from build123d import *

# Parameters (mm, degrees)
SKETCH1_W           = 27
SKETCH1_H           = 50
BOSS_EXTRUDE1_DEPTH = 4.5
SKETCH2_W           = 8.18
SKETCH2_H           = 8.18
BOSS_EXTRUDE2_DEPTH = 6.7
SKETCH3_R           = 0.8
CUT_EXTRUDE1_DEPTH  = 6.7


with BuildPart() as part:
    # Sketch1 → Boss-Extrude1 (new body)
    with BuildSketch(Plane.XY):
        Rectangle(SKETCH1_W, SKETCH1_H)
    extrude(amount=BOSS_EXTRUDE1_DEPTH)

    # Sketch2 → Boss-Extrude2 (add)
    with BuildSketch(Plane.XY.offset(4.5)):
        with Locations((0, 18)):
            Rectangle(SKETCH2_W, SKETCH2_H)
    extrude(amount=BOSS_EXTRUDE2_DEPTH)

    # Sketch3 → Cut-Extrude1 (cut)
    with BuildSketch(Plane.XY.offset(4.5)):
        with Locations((10.7092899, 15.271061343)):
            Circle(SKETCH3_R)
        with Locations((10.7092899, 12.271061343)):
            Circle(SKETCH3_R)
        with Locations((10.7092899, 9.271061343)):
            Circle(SKETCH3_R)
        with Locations((10.7092899, 6.271061343)):
            Circle(SKETCH3_R)
        with Locations((10.7092899, 3.271061343)):
            Circle(SKETCH3_R)
        with Locations((10.7092899, 0.271061343)):
            Circle(SKETCH3_R)
        with Locations((10.7092899, -2.728938657)):
            Circle(SKETCH3_R)
        with Locations((10.7092899, -5.728938657)):
            Circle(SKETCH3_R)
        with Locations((10.7092899, -8.728938657)):
            Circle(SKETCH3_R)
        with Locations((10.7092899, -11.728938657)):
            Circle(SKETCH3_R)
    cut_extrude1 = extrude(amount=-CUT_EXTRUDE1_DEPTH, mode=Mode.SUBTRACT)

    # Mirror1: Cut-Extrude1 across plane
    add(cut_extrude1.mirror(Plane(origin=(0, 0, 0), x_dir=(0, 0, 1), z_dir=(1, 0, 0))), mode=Mode.SUBTRACT)


solid = part.part
The model under review builds one solid part; all positions refer to its coordinate system, in mm. A direction names the side the tool comes from. Round coordinates to 2 decimals unless told otherwise and drop trailing zeros. Loops run counter-clockwise (first coordinate to the right, second up) from the corner with the lowest first, then second, coordinate; pieces in that order, holes last. Notation, with made-up numbers: (88, 28) -> (126, 28) arc R17 ccw to (126, 48) -> close; hole circle Ø10 at (12.5, -8). An arc over 180 degrees is marked (long way). Return JSON: item names as keys, results as strings.
(1) For faces 1 (the cylindrical face through (11.448, -9.035, 2.282)), 2 (the flat face through (0, 22.09, 8)), 3 (the flat face through (4.09, 18, 8)), list the 3-axis set-ups (+Z, -Z, +X, -X, +Y, -Y) from which the entire face can be reached by the end or side of a thin tool; tool diameter is ignored.
Solved:
{"face 1": "+Z, -Z", "face 2": "+Z, +X, -X, +Y", "face 3": "+Z, +X, +Y, -Y"}
(2) Add section B-B on x = 2.5. Write out the cut boundary in (y, z).
Solved:
{"outline": "(-25, 0) -> (25, 0) -> (25, 4.5) -> (22.09, 4.5) -> (22.09, 11.2) -> (13.91, 11.2) -> (13.91, 4.5) -> (-25, 4.5) -> close"}
(3) Add section A-A on z = 3.75. State how many separate pieces and enclosed holes the cut face has, plus the area to 3 significant figures.
Solved:
{"separate pieces": "1", "enclosed holes": "20", "area": "1,310 mm2"}
(4) For pin 1 (4 mm diameter, centred on x = 0, z = 9.5, fed in from +Y); pin 2 (1 mm diameter, centred on x = 10.71, y = 3.27, fed in from -Z); pin 3 (2.5 mm diameter, centred on x = -10.71, y = 0.27, fed in from +Z); pin 4 (5.5 mm diameter, centred on y = 17, z = 9, fed in from -X), all flat-tipped, find the tip position at first contact; note any pin that passes through.
Solved:
{"pin 1": "y = 22.09", "pin 2": "through", "pin 3": "z = 4.5", "pin 4": "x = -4.09"}
(5) Add section C-C on y = -20. Write out the cut boundary in (x, z), plus the area to 4 significant figures.
Solved:
{"outline": "(-13.5, 0) -> (13.5, 0) -> (13.5, 4.5) -> (-13.5, 4.5) -> close", "area": "121.5 mm2"}
(6) The part is to be moulded in two halves that separate along X. For faces 4 (the flat face through (13.5, 0, 2)), 5 (the flat face through (0, 13.91, 8)), 6 (the cylindrical face through (11.472, -2.489, 2.282)), say which applies: released by +X, released by -X, zero draft, split by the parting line, or undercut.
Solved:
{"face 4": "released by +X", "face 5": "zero draft", "face 6": "undercut"}
(7) For line 1 (Z direction, x = 3.5, y = -5); line 2 (Y direction, x = 0.5, z = 7); line 3 (X direction, y = 16, z = 7), list the stretches that pass through material, from the lowest coordinate up.
Solved:
{"line 1": "0 to 4.5", "line 2": "13.91 to 22.09", "line 3": "-4.09 to 4.09"}
(8) Add section D-D on z = 8.75. Write out the cut boundary in (x, y), plus the area to 3 significant figures.
Solved:
{"outline": "(-4.09, 13.91) -> (4.09, 13.91) -> (4.09, 22.09) -> (-4.09, 22.09) -> close", "area": "66.9 mm2"}
